```python
from build123d import *

# Parameters (mm, degrees)
SKETCH_1_R          = 11.555
EXTRUDE_1_DEPTH     = 11
SKETCH_2_R          = 14
EXTRUDE_2_DEPTH     = 2
EXTRUDE_START       = 2
SKETCH_3_R          = 14
EXTRUDE_3_DEPTH     = 2
SKETCH_4_R          = 2.5
CUT_EXTRUDE_1_DEPTH = 25.839484697


with BuildPart() as part:
    # 草图1 → 凸台-拉伸1 (new body)
    with BuildSketch(Plane.XY):
        Circle(SKETCH_1_R)
    extrude(amount=EXTRUDE_1_DEPTH)

    # 草图2 → 凸台-拉伸2 (add)
    with BuildSketch(Plane.XY.offset(11)):
        Circle(SKETCH_2_R)
    extrude(amount=EXTRUDE_2_DEPTH)

    # 草图3 → 凸台-拉伸3 (add)
    with BuildSketch(Plane(origin=(0, 0, 0), x_dir=(-1, 0, 0), z_dir=(0, 0, -1)).offset(EXTRUDE_START)):
        with Locations(Location((0, 0, 0), (0, 0, 180))):
            Circle(SKETCH_3_R)
    extrude(amount=-EXTRUDE_3_DEPTH)

    # 草图4 → 切除-拉伸1 (cut, through all)
    with BuildSketch(Plane(origin=(0, 0, -2), x_dir=(-1, 0, 0), z_dir=(0, 0, -1))):
        Circle(SKETCH_4_R)
    extrude(amount=-CUT_EXTRUDE_1_DEPTH, mode=Mode.SUBTRACT)


solid = part.part
```
Here's how the part is built. I have some questions about the finished solid (model axes, mm). A direction names the side the tool comes from. Coordinates: 2 decimals unless noted, no trailing zeros. Order: outer loops, then holes, each group sorted by start corner. A loop starts at its lowest first (then second) coordinate and runs counter-clockwise, first axis right, second up. Notation, with made-up numbers: (-28, 77) -> (-18, 77) arc R25 ccw to (-18, 111) -> close; hole circle Ø11 at (73.5, 11.25). An arc over 180 degrees is marked (long way). Return JSON: item names as keys, results as strings.
1) If we section it at D-D on x = -4.25: List the corners of the cut face in (y, z) for me, plus the area to 3 significant figures.
Conclusion:
{"outline": "(-13.34, -2) -> (13.34, -2) -> (13.34, 0) -> (10.75, 0) -> (10.75, 11) -> (13.34, 11) -> (13.34, 13) -> (-13.34, 13) -> (-13.34, 11) -> (-10.75, 11) -> (-10.75, 0) -> (-13.34, 0) -> close", "area": "343 mm²"}
2) Thinking about a two-plate mould opening in Z: for faces 3 (the flat face through (-3.2, 11.5, 11)), 4 (the flat face through (3, 0, 13)), 5 (the flat face through (3, 0, -2)), which applies, +Z half, -Z half, draft (parallel to the pull), parting line (faces both ways), or undercut?
Conclusion:
{"face 3": "undercut", "face 4": "+Z half", "face 5": "-Z half"}
3) If I drill on probe 1 along Y at (x, z) = (0, 3.75) (3 decimals); probe 2 along Z at (x, y) = (-7.5, 11.25); probe 3 along X at (y, z) = (-2, 10.75), over which ranges is the centre line in solid material (lowest first)?
Conclusion:
{"probe 1": "y = -11.555 to -2.5, 2.5 to 11.555", "probe 2": "z = -2 to 0, 11 to 13", "probe 3": "x = -11.38 to -1.5, 1.5 to 11.38"}
4) If we section it at C-C on z = 7.75: List the corners of the cut face in (x, y) for me (3 decimals).
Conclusion:
{"outline": "circle Ø23.11 at (0, 0); hole circle Ø5 at (0, 0)"}
5) If we section it at A-A on y = 0: List the corners of the cut face in (x, z) for me (3 decimals).
Conclusion:
{"outline": "(-14, -2) -> (-2.5, -2) -> (-2.5, 13) -> (-14, 13) -> (-14, 11) -> (-11.555, 11) -> (-11.555, 0) -> (-14, 0) -> close; (2.5, -2) -> (14, -2) -> (14, 0) -> (11.555, 0) -> (11.555, 11) -> (14, 11) -> (14, 13) -> (2.5, 13) -> close"}
6) I'm going to push flat-ended pins straight in: P1, Ø4, axis at y = 0.5, z = 4.5, coming from the +X side (3 decimals); P2, Ø8, axis at x = -5.5, z = 3.5, coming from the +Y side; P3, Ø6, axis at y = 4, z = 3.5, coming from the +X side. Where does each tip first touch, or does it pass through?
Conclusion:
{"P1": "stops at x = 11.555", "P2": "stops at y = 13.54", "P3": "stops at x = 11.51"}
7) On a 3-axis mill with a long thin cutter (end or side, diameter ignored), from which of +Z, -Z, +X, -X, +Y, -Y can I reach the whole of each face in a straight line? I mean faces 1 (the flat face through (-3.2, -11.5, 0)), 2 (the cylindrical face through (0.54, -2.44, 5.4)). Say none if no direction works.
Conclusion:
{"face 1": "none", "face 2": "+Z, -Z"}
